Input: dimensioned drawing with shaded views. Units: mm. Origin: part minimum x, y, z. Round coordinates to 2 decimals unless told otherwise and drop trailing zeros. Write each loop counter-clockwise with the first axis right and the second up, starting at its lowest first coordinate (ties: lowest second). Pieces come first, ordered by that corner, then holes. Notation, with made-up numbers: (28.25, 38) - (50.25, 38) arc R7 cw to (50.25, 44) - close; hole circle Ø1 at (88.5, 18.5). An arc over 180 degrees is marked (long way). Use one line per item in the form item = value.
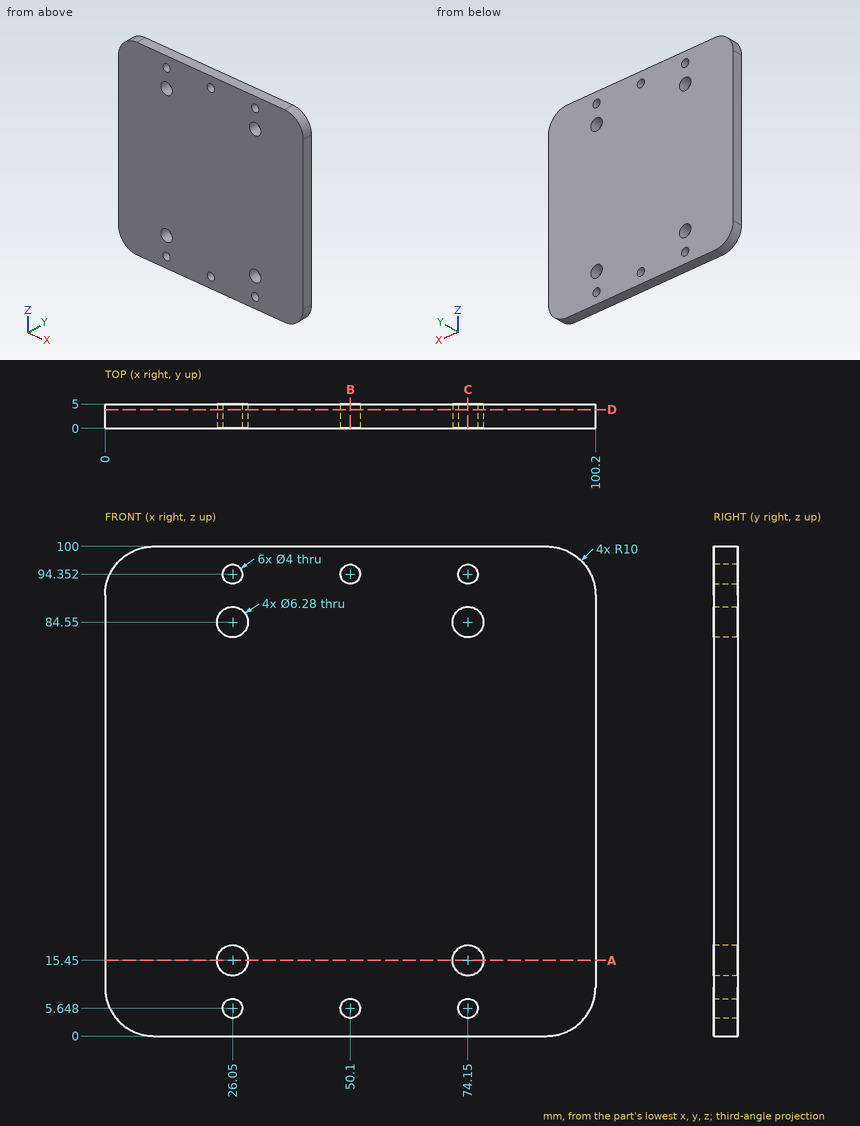
(1) Cut plane B-B on x = 50.1. Output: boundary loops of the cut face in (y, z).
Derived:
outline = (0, 0) - (5, 0) - (5, 3.65) - (0, 3.65) - close; (0, 7.65) - (5, 7.65) - (5, 92.35) - (0, 92.35) - close; (0, 96.35) - (5, 96.35) - (5, 100) - (0, 100) - close
(2) Cut plane C-C on x = 74.15. Output: boundary loops of the cut face in (y, z).
Derived:
outline = (0, 0) - (5, 0) - (5, 3.65) - (0, 3.65) - close; (0, 7.65) - (5, 7.65) - (5, 12.31) - (0, 12.31) - close; (0, 18.59) - (5, 18.59) - (5, 81.41) - (0, 81.41) - close; (0, 87.69) - (5, 87.69) - (5, 92.35) - (0, 92.35) - close; (0, 96.35) - (5, 96.35) - (5, 100) - (0, 100) - close
(3) Material intervals for L1, parallel to X at y = 3.5, z = 84.55; L2, parallel to X at y = 2.85, z = 18 (1 decimal); L3, parallel to X at y = 1.95, z = 8, sorted ascending.
Derived:
L1 = 0 to 22.91, 29.19 to 71.01, 77.29 to 100.2
L2 = 0 to 24.2, 27.9 to 72.3, 76 to 100.2
L3 = 0.2 to 100
(4) Cut plane A-A on z = 15.45. Output: boundary loops of the cut face in (x, y).
Derived:
outline = (0, 0) - (22.91, 0) - (22.91, 5) - (0, 5) - close; (29.19, 0) - (71.01, 0) - (71.01, 5) - (29.19, 5) - close; (77.29, 0) - (100.2, 0) - (100.2, 5) - (77.29, 5) - close
(5) First-contact query: pin 1 Ø5 at (x, z) = (26.05, 94.35) entering from -Y. Flat tip, straight axial feed; report the tip coordinate or a pass-through.
Derived:
pin_1 = 0
(6) Cut plane D-D on y = 3.85. Count the separate pieces of the cut face and the enclosed holes in it.
Derived:
separate_pieces = 1
enclosed_holes = 10
